```python
from build123d import *

# Parameters (mm, degrees)
F0_W     = 76.2
F0_H     = 21.59
F1_DEPTH = 5.08
F2_W     = 2.54
F2_H     = 21.59
F3_DEPTH = 3.81
F5_DEPTH = 25.4
F7_DEPTH = 21.59


# Not quite as in the source:
# - a feature names something its author has since deleted; it is built from what else it names


with BuildPart() as f1:
    # F0 (on Top) → F1 (new body)
    with BuildSketch(Plane.XY):
        with Locations((38.1, 10.795)):
            Rectangle(F0_W, F0_H)
    extrude(amount=F1_DEPTH)

    # F2 (on face) → F3 (join)
    with BuildSketch(Plane.XY.offset(5.08)):
        with Locations((1.27, 10.795)):
            Rectangle(F2_W, F2_H)
        with Locations((74.93, 10.795)):
            Rectangle(F2_W, F2_H)
    extrude(amount=F3_DEPTH)

    # F4 (on face) → F5 (cut)
    with BuildSketch(Plane.XY.offset(5.08)):
        with BuildLine():
            ThreePointArc((29.21, 21.59), (38.1, 12.7), (46.99, 21.59))
            Line((46.99, 21.59), (29.21, 21.59))
        make_face()
        with BuildLine():
            Line((29.21, 21.59), (46.99, 21.59))
            ThreePointArc((46.99, 21.59), (38.1, 30.48), (29.21, 21.59))
        make_face()
    extrude(amount=-F5_DEPTH, mode=Mode.SUBTRACT)

    # F6 (on face) → F7 (join, through all)
    with BuildSketch(Plane.XZ):
        Polygon((0, 5.08), (0, 8.89), (-1.27, 8.89), align=None)
        Polygon((76.2, 8.89), (76.2, 5.08), (77.47, 8.89), align=None)
    extrude(amount=-F7_DEPTH)


solid = f1.part
```
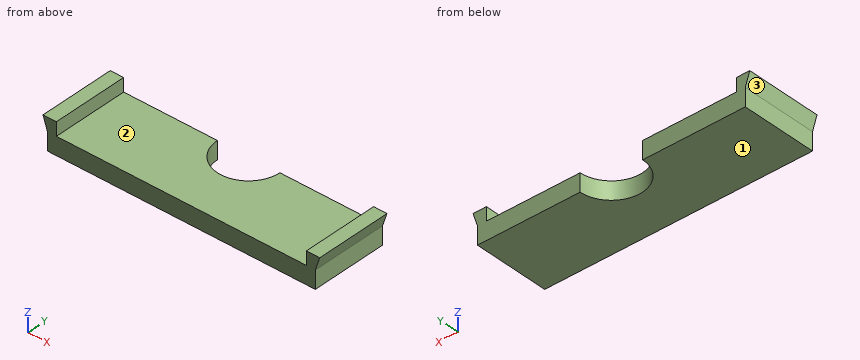
The listing builds one solid part. Answer for the finished solid, in the listing's coordinates (mm). Face numbers are marked on the shaded views. Coordinates: 2 decimals unless noted, no trailing zeros. Loops run counter-clockwise (first coordinate to the right, second up) from the corner with the lowest first, then second, coordinate; pieces in that order, holes last. Notation, with made-up numbers: (-5, -14.75) -> (40, -14.75) arc R30 ccw to (40, 11.25) -> close; hole circle Ø1 at (2, -8.75). An arc over 180 degrees is marked (long way). Return JSON: item names as keys, results as strings. Group by question number.
(1) A cutting plane is placed at A-A on z = 6. Write down the section's boundary in (x, y), and give its area (3 significant figures).
(2) A cutting plane is placed at C-C on y = 15.75. Write down the section's boundary in (x, z), and give its area (3 significant figures).
(3) Find the intervals of material crossed by probe 1 along X at (y, z) = (12.25, 5); probe 2 along Z at (x, y) = (57.5, 6.5); probe 3 along X at (y, z) = (18.5, 5.25), in increasing order. Write a range as from..to.
(4) A cutting plane is placed at B-B on y = 9.5. Write down the section's boundary in (x, z), and give its area (3 significant figures).
(5) Given pin 1 Ø1 at (y, z) = (12, 2) entering from +X; pin 2 Ø2 at (y, z) = (15.5, 1) entering from -X; pin 3 Ø5 at (x, z) = (56, 6.5) entering from -Y; pin 4 Ø8 at (x, y) = (25, 18) entering from +Z, each flat-ended and moving along its own axis, determine where each tip first touches the part or whether it passes through.
(6) Determine the mould class of the marked faces 1, 2 and 3 for opening direction X: released by +X, released by -X, zero draft, split by the parting line, or undercut.
(7) A cutting plane is placed at D-D on x = 38.1. Write down the section's boundary in (y, z).
The answers:
{
 "1": {"outline": "(-0.31, 0) -> (2.54, 0) -> (2.54, 21.59) -> (-0.31, 21.59) -> close; (73.66, 0) -> (76.51, 0) -> (76.51, 21.59) -> (73.66, 21.59) -> close", "area": "123 mm^2"},
 "2": {"outline": "(-1.27, 8.89) -> (0, 5.08) -> (0, 0) -> (31.4, 0) -> (31.4, 5.08) -> (2.54, 5.08) -> (2.54, 8.89) -> close; (44.8, 0) -> (76.2, 0) -> (76.2, 5.08) -> (77.47, 8.89) -> (73.66, 8.89) -> (73.66, 5.08) -> (44.8, 5.08) -> close", "area": "343 mm^2"},
 "3": {"probe 1": "x = 0..76.2", "probe 2": "z = 0..5.08", "probe 3": "x = -0.06..2.54, 73.66..76.26"},
 "4": {"outline": "(-1.27, 8.89) -> (0, 5.08) -> (0, 0) -> (76.2, 0) -> (76.2, 5.08) -> (77.47, 8.89) -> (73.66, 8.89) -> (73.66, 5.08) -> (2.54, 5.08) -> (2.54, 8.89) -> close", "area": "411 mm^2"},
 "5": {"pin 1": "stops at x = 76.2", "pin 2": "stops at x = 0", "pin 3": "stops at y = 0", "pin 4": "stops at z = 5.08"},
 "6": {"face 1": "zero draft", "face 2": "undercut", "face 3": "released by -X"},
 "7": {"outline": "(0, 0) -> (12.7, 0) -> (12.7, 5.08) -> (0, 5.08) -> close"}
}
